Input: part model. Units: mm. Frame: model coordinates. A direction names the side the tool comes from. Round coordinates to 2 decimals unless told otherwise and drop trailing zeros. Loops run counter-clockwise (first coordinate to the right, second up) from the corner with the lowest first, then second, coordinate; pieces in that order, holes last. Notation, with made-up numbers: (-20, 66) - (36, 66) arc R24 ccw to (36, 101) - close; hole circle Ø5 at (-40, 38.5). An arc over 180 degrees is marked (long way). Use CSV: the item, a comma, the result in double quotes. Start each with the question number.
1. Material intervals for probe 1 along Y at (x, z) = (-12, 6.25); probe 2 along X at (y, z) = (4.75, 7.5); probe 3 along Y at (x, z) = (-1.75, 6), sorted ascending. Write a range as from..to.
2. Pull-direction query (Y, two-part tool) for faces 4 (the flat face through (-9, 4.9, 5)), 5 (the flat face through (-8, 0, 5)), 6 (the flat face through (-15, 4, 5)); classes: +Y half, -Y half, draft (parallel to the pull), parting line (faces both ways), or undercut.
3. Cut plane B-B (z = 4.5). Return loops of the section in (x, y).
4. Cut plane C-C (x = -9.25). Return loops of the section in (y, z), and give its area (3 significant figures).
5. Cut plane D-D (y = 1.75). Return loops of the section in (x, z), and give its area (3 significant figures).
6. Access query for faces 1 (the flat face through (0, 10, 5)), 2 (the flat face through (-8, 2.9, 5)), 3 (the flat face through (2, 5, 5)). Directions: +Z, -Z, +X, -X, +Y, -Y. A direction counts if a zero-diameter tool reaches every point of the face in a straight line with its end or side. Return the directions, or none.
7. Pin query (flat end, axial travel): P1, Ø0.9, axis at y = 1, z = 5.5, coming from the -X side; P2, Ø8, axis at x = -12.5, y = 1.5, coming from the -Z side; P3, Ø3, axis at x = -11, z = 3.5, coming from the +Y side; P4, Ø0.6, axis at y = 4, z = 4, coming from the -X side. Return the tip coordinate at first contact, or that it passes through.
8. Cut plane A-A (x = -2.5). Return loops of the section in (y, z), and give its area (3 significant figures).
```python
from build123d import *

# Parameters (mm, degrees)
F0_W     = 15.193479
F0_H     = 2
F1_DEPTH = 10


with BuildPart() as f1:
    # F0 (on Top) → F1 (new body)
    with BuildSketch(Plane.XY):
        with Locations((-7.596739, -1)):
            Rectangle(F0_W, F0_H)
        with BuildLine():
            Line((0, 2.9), (0, 0))
            Line((0, 0), (0, -2))
            Line((0, -2), (2, -2))
            Line((2, -2), (2, 13))
            Line((2, 13), (0, 13))
            Line((0, 13), (0, 7.9))
            ThreePointArc((0, 7.9), (-0.87868, 5.77868), (-3, 4.9))
            Line((-3, 4.9), (-15, 4.9))
            Line((-15, 4.9), (-15, 2.9))
            Line((-15, 2.9), (0, 2.9))
        make_face()
    extrude(amount=F1_DEPTH)


solid = f1.part
```
Established:
1,probe 1,"y = -2..0, 2.9..4.9"
1,probe 2,"x = -15..2"
1,probe 3,"y = -2..0, 2.9..5.17"
2,face 4,"+Y half"
2,face 5,"undercut"
2,face 6,"draft"
3,outline,"(-15.19, -2) - (2, -2) - (2, 13) - (0, 13) - (0, 7.9) arc R3 cw to (-3, 4.9) - (-15, 4.9) - (-15, 2.9) - (0, 2.9) - (0, 0) - (-15.19, 0) - close"
4,outline,"(-2, 0) - (0, 0) - (0, 10) - (-2, 10) - close; (2.9, 0) - (4.9, 0) - (4.9, 10) - (2.9, 10) - close"
4,area,"40.0 mm2"
5,outline,"(0, 0) - (2, 0) - (2, 10) - (0, 10) - close"
5,area,"20.0 mm2"
6,face 1,"+Z, -Z, -X, +Y"
6,face 2,"+Z, -Z, -X"
6,face 3,"+Z, -Z, +X, +Y, -Y"
7,P1,"stops at x = 0"
7,P2,"stops at z = 0"
7,P3,"stops at y = 4.9"
7,P4,"stops at x = -15"
8,outline,"(-2, 0) - (0, 0) - (0, 10) - (-2, 10) - close; (2.9, 0) - (4.94, 0) - (4.94, 10) - (2.9, 10) - close"
8,area,"40.4 mm2"
